Design review of the part built by this model. Coordinates are the model's own, in mm. Face numbers are marked on the shaded views. A direction names the side the tool comes from. Give positions to 0.01 mm unless a question says otherwise; leave off trailing zeros. Write each loop counter-clockwise with the first axis right and the second up, starting at its lowest first coordinate (ties: lowest second). Pieces come first, ordered by that corner, then holes. Notation, with made-up numbers: (68.5, 27.5) -> (87.5, 27.5) arc R9 ccw to (87.5, 37.5) -> close; hole circle Ø7 at (-21.75, 40.5). An arc over 180 degrees is marked (long way). Put each result on its own line as item: value. Start each with the question number.
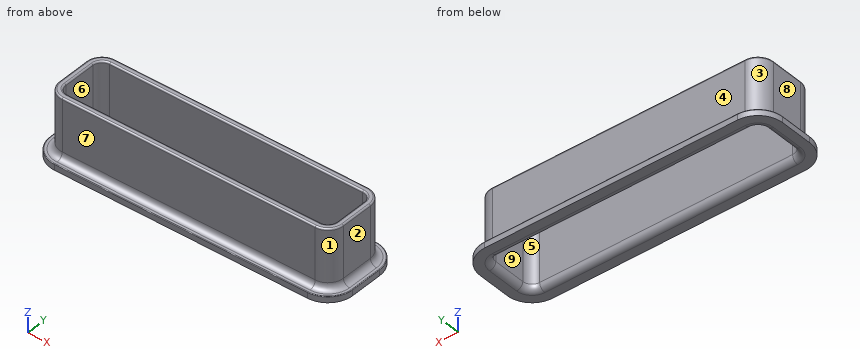
from build123d import *

# Parameters (mm, degrees)
BOSS_EXTRUDE1_DEPTH = 2
BOSS_EXTRUDE2_DEPTH = 19
CUT_EXTRUDE1_DEPTH  = 32
FILLET1_R           = 0.5
FILLET2_R           = 2
FILLET3_R           = 2
FILLET4_R           = 0.2


with BuildPart() as part:
    # Sketch1 → Boss-Extrude1 (new body)
    with BuildSketch(Plane.XY):
        with BuildLine():
            Line((-1.128427562, 10.874070422), (80.75048871, 10.874070422))
            ThreePointArc((80.75048871, 10.874070422), (86.40734296, 8.530924671), (88.75048871, 2.874070422))
            Line((88.75048871, 2.874070422), (88.75048871, -7.709925539))
            ThreePointArc((88.75048871, -7.709925539), (86.40734296, -13.366779789), (80.75048871, -15.709925539))
            Line((80.75048871, -15.709925539), (-1.128427562, -15.709925539))
            ThreePointArc((-1.128427562, -15.709925539), (-6.785281811, -13.366779789), (-9.128427562, -7.709925539))
            Line((-9.128427562, -7.709925539), (-9.128427562, 2.874070422))
            ThreePointArc((-9.128427562, 2.874070422), (-6.785281811, 8.530924671), (-1.128427562, 10.874070422))
        make_face()
    extrude(amount=-BOSS_EXTRUDE1_DEPTH)

    # Sketch1_6 → Boss-Extrude2 (add)
    with BuildSketch(Plane.XY):
        with BuildLine():
            Line((-1.128427562, 7.874070422), (80.75048871, 7.874070422))
            ThreePointArc((80.75048871, 7.874070422), (84.286022616, 6.409604328), (85.75048871, 2.874070422))
            Line((85.75048871, 2.874070422), (85.75048871, -7.709925539))
            ThreePointArc((85.75048871, -7.709925539), (84.286022616, -11.245459445), (80.75048871, -12.709925539))
            Line((80.75048871, -12.709925539), (-1.128427562, -12.709925539))
            ThreePointArc((-1.128427562, -12.709925539), (-4.663961468, -11.245459445), (-6.128427562, -7.709925539))
            Line((-6.128427562, -7.709925539), (-6.128427562, 2.874070422))
            ThreePointArc((-6.128427562, 2.874070422), (-4.663961468, 6.409604328), (-1.128427562, 7.874070422))
        make_face()
    extrude(amount=BOSS_EXTRUDE2_DEPTH)

    # Sketch2 → Cut-Extrude1 (cut)
    with BuildSketch(Plane.XY.offset(19)):
        with BuildLine():
            Line((-4.128427562, 2.874070422), (-4.128427562, -7.709925539))
            ThreePointArc((-4.128427562, -7.709925539), (-3.249747905, -9.831245883), (-1.128427562, -10.709925539))
            Line((-1.128427562, -10.709925539), (80.75048871, -10.709925539))
            ThreePointArc((80.75048871, -10.709925539), (82.871809054, -9.831245883), (83.75048871, -7.709925539))
            Line((83.75048871, -7.709925539), (83.75048871, 2.874070422))
            ThreePointArc((83.75048871, 2.874070422), (82.871809054, 4.995390765), (80.75048871, 5.874070422))
            Line((80.75048871, 5.874070422), (-1.128427562, 5.874070422))
            ThreePointArc((-1.128427562, 5.874070422), (-3.249747905, 4.995390765), (-4.128427562, 2.874070422))
        make_face()
    extrude(amount=-CUT_EXTRUDE1_DEPTH, mode=Mode.SUBTRACT)

    # Fillet1
    fillet1_edges = [part.edges().sort_by_distance(p)[0] for p in [
        (-4.663961468, 6.409604328, 19),
        (-4.663961468, -11.245459445, 19),
        (84.286022616, -11.245459445, 19),
        (85.75048871, -2.417927559, 19),
        (84.286022616, 6.409604328, 19),
        (39.811030574, 7.874070422, 19),
        (-6.128427562, -2.417927559, 19),
        (39.811030574, -12.709925539, 19),
        (-3.249747905, 4.995390765, 19),
        (-4.128427562, -2.417927559, 19),
        (-3.249747905, -9.831245883, 19),
        (39.811030574, -10.709925539, 19),
        (82.871809054, -9.831245883, 19),
        (83.75048871, -2.417927559, 19),
        (82.871809054, 4.995390765, 19),
        (39.811030574, 5.874070422, 19),
    ]]
    fillet(fillet1_edges, radius=FILLET1_R)

    # Fillet2
    fillet2_edges = [part.edges().sort_by_distance(p)[0] for p in [
        (-6.128427562, -2.417927559, 0),
        (39.811030574, -12.709925539, 0),
        (-4.663961468, 6.409604328, 0),
        (39.811030574, 7.874070422, 0),
        (84.286022616, 6.409604328, 0),
        (85.75048871, -2.417927559, 0),
        (84.286022616, -11.245459445, 0),
        (-4.663961468, -11.245459445, 0),
    ]]
    fillet(fillet2_edges, radius=FILLET2_R)

    # Fillet3
    fillet3_edges = [part.edges().sort_by_distance(p)[0] for p in [
        (-3.249747905, 4.995390765, -2),
        (39.811030574, 5.874070422, -2),
        (82.871809054, 4.995390765, -2),
        (83.75048871, -2.417927559, -2),
        (82.871809054, -9.831245883, -2),
        (39.811030574, -10.709925539, -2),
        (-3.249747905, -9.831245883, -2),
        (-4.128427562, -2.417927559, -2),
    ]]
    fillet(fillet3_edges, radius=FILLET3_R)

    # Fillet4
    fillet4_edges = [part.edges().sort_by_distance(p)[0] for p in [
        (86.40734296, 8.530924671, 0),
        (88.75048871, -2.417927559, 0),
        (86.40734296, -13.366779789, 0),
        (39.811030574, -15.709925539, 0),
        (-6.785281811, -13.366779789, 0),
        (-9.128427562, -2.417927559, 0),
        (-6.785281811, 8.530924671, 0),
        (39.811030574, 10.874070422, 0),
    ]]
    fillet(fillet4_edges, radius=FILLET4_R)


solid = part.part
Q1. Machinability: for the marked faces 1, 2, 3, 4 and 5, which of the approach directions +Z, -Z, +X, -X, +Y, -Y give a long, thin tool a straight path to every point of the face, cutting with its end or side? Answer none if there is none.
Q2. To check wall thickness, follow probe 1 along X at (y, z) = (2, 3); probe 2 along Y at (x, z) = (13, 11.25). State the ranges of each line that lie inside material, in increasing order. Write a range as from..to.
Q3. Mouldability with a two-part tool opening along X and no side actions: class the marked faces 6, 7, 8 and 9 as +X half, -X half, draft (parallel to the pull), parting line (faces both ways), or undercut.
Q4. Take a section at B-B on x = 5.5. Give the boundary of the cut face in (y, z), then the cut area to 3 significant figures.
Q5. Take a section at A-A on z = 4.75. Give the boundary of the cut face in (x, y), then the cut area to 3 significant figures.
Q6. For pin 1 (10 mm diameter, centred on x = 32.5, z = 9.5, fed in from -Y); pin 2 (8 mm diameter, centred on x = 7.5, z = 16.5, fed in from +Y); pin 3 (11.5 mm diameter, centred on y = -2.5, z = 6.5, fed in from +X), all flat-tipped, find the tip position at first contact; note any pin that passes through.
Result:
1. face 1: +Z, +X, -Y
1. face 2: +Z, +X, +Y, -Y
1. face 3: +Z, -X, +Y
1. face 4: +Z, +X, -X, +Y
1. face 5: +Z, -Z
2. probe 1: x = -6.13..-4.13, 83.75..85.75
2. probe 2: y = -12.71..-10.71, 5.87..7.87
3. face 6: undercut
3. face 7: draft
3. face 8: -X half
3. face 9: undercut
4. outline: (-15.71, -2) -> (-12.71, -2) arc R2 ccw to (-10.71, 0) -> (-10.71, 18.5) arc R0.5 ccw to (-11.21, 19) -> (-12.21, 19) arc R0.5 ccw to (-12.71, 18.5) -> (-12.71, 2) arc R2 cw to (-14.71, 0) -> (-15.51, 0) arc R0.2 ccw to (-15.71, -0.2) -> close; (5.87, 0) arc R2 ccw to (7.87, -2) -> (10.87, -2) -> (10.87, -0.2) arc R0.2 ccw to (10.67, 0) -> (9.87, 0) arc R2 cw to (7.87, 2) -> (7.87, 18.5) arc R0.5 ccw to (7.37, 19) -> (6.37, 19) arc R0.5 ccw to (5.87, 18.5) -> close
4. area: 95.8 mm^2
5. outline: (-6.13, -7.71) arc R5 ccw to (-1.13, -12.71) -> (80.75, -12.71) arc R5 ccw to (85.75, -7.71) -> (85.75, 2.87) arc R5 ccw to (80.75, 7.87) -> (-1.13, 7.87) arc R5 ccw to (-6.13, 2.87) -> close; hole (-4.13, -7.71) arc R3 ccw to (-1.13, -10.71) -> (80.75, -10.71) arc R3 ccw to (83.75, -7.71) -> (83.75, 2.87) arc R3 ccw to (80.75, 5.87) -> (-1.13, 5.87) arc R3 ccw to (-4.13, 2.87) -> close
5. area: 420 mm^2
6. pin 1: stops at y = -12.71
6. pin 2: stops at y = 7.87
6. pin 3: stops at x = 86.19
